For this review, take the finished solid that the model builds, in its own axes (mm). A direction names the side the tool comes from. Round coordinates to 2 decimals unless told otherwise and drop trailing zeros. Write each loop counter-clockwise with the first axis right and the second up, starting at its lowest first coordinate (ties: lowest second). Pieces come first, ordered by that corner, then holes. Notation, with made-up numbers: (46, -6) - (54, -6) arc R23 ccw to (54, 18) - close; hole circle Ø2 at (15.5, 68.25). An arc over 180 degrees is marked (long way). One line per item, written item: value. Start each with the question number.
Q1. Tool access review of faces 4 (the face through (-2.019, -46, 3)), 5 (the face through (24.11, -21.92, 2.96)), 6 (the face through (21.81, -25.64, 2.96)): name each direction out of +Z, -Z, +X, -X, +Y, -Y from which nothing blocks a thin tool from reaching the whole face with its end or side.
Q2. For probe 1 along Y at (x, z) = (-6, 1.75); probe 2 along X at (y, z) = (-29.5, 3.25); probe 3 along X at (y, z) = (-23.25, 2.2), list the stretches that pass through material, from the lowest coordinate up.
Q3. Add section A-A on x = 25. Write out the cut boundary in (y, z), and give its area (3 significant figures).
Q4. Add section B-B on z = 0.6. Give the number of separate pieces and of enclosed holes in the cut face, and give its area (3 significant figures).
Q5. Add section D-D on x = 9. Write out the cut boundary in (y, z), and give its area (3 significant figures).
Q6. Clearance check with flat-ended pins moving along their axes: pin 1 Ø2.5 at (x, y) = (25.18, -44.68) entering from -Z; pin 2 Ø4 at (x, y) = (4, -26) entering from +Z. State where each tip first meets the part, or that it passes through.
Q7. Add section C-C on y = -38. Write out the cut boundary in (x, z).
Q8. Mouldability with a two-part tool opening along Y and no side actions: class faces 1 (the face through (-1.449, -41.785, 2.958)), 2 (the face through (10, -34, 0)), 3 (the face through (1.5, -30.38, 2.96)) as +Y half, -Y half, draft (parallel to the pull), parting line (faces both ways), or undercut.
Autodesk Inventor part; units mm, degrees
ref_plane "YZ Plane" through (0, 0, 0) normal (1, 0, 0) x (0, 1, 0)
ref_plane "XZ Plane" through (0, 0, 0) normal (0, 1, 0) x (-1, 0, 0)
ref_plane "XY Plane" through (0, 0, 0) normal (0, 0, 1) x (1, 0, 0)
sketch "스케치1" plane through (0, 0, 0) normal (0, 0, 1) x (1, 0, 0)
  line L0 (22.3806, -23.2436) -> (22.3806, 15.7564)
  arc A0 (20.3806, -26.2436) -> (22.3806, -24.2436) centre (20.3806, -24.2436) ccw
  line L1 (22.3806, -24.2436) -> (22.3806, -22.8439)
  line L2 (18.7808, -26.2436) -> (20.3806, -26.2436)
  line L3 (0.9806, -26.2436) -> (19.3806, -26.2436)
  arc A1 (-2.0194, -24.2436) -> (-0.0194, -26.2436) centre (-0.0194, -24.2436) ccw
  line L4 (-0.0194, -26.2436) -> (1.5803, -26.2436)
  line L5 (-2.0194, -24.2436) -> (-2.0194, -22.8439)
  line L6 (-2.0194, 15.7564) -> (-2.0194, -23.2436)
  circle A2 centre (25.1806, -22.7436) radius 1.45
  circle A3 centre (18.6806, -29.0436) radius 1.45
  circle A4 centre (1.6806, -29.0436) radius 1.45
  circle A5 centre (-4.8194, -22.7436) radius 1.45
  line L7 (-7.6194, -18.7138) -> (27.9806, -18.7138)
  line L8 (-7.6194, -18.7138) -> (27.9806, -18.7138)
  arc A6 (-0.0194, -41.1839) -> (-2.0194, -43.1839) centre (-0.0194, -43.1839) ccw
  line L9 (-2.0194, -43.1839) -> (-2.0194, -44.5837)
  line L10 (1.5803, -41.1839) -> (-0.0194, -41.1839)
  line L11 (19.3806, -41.1839) -> (0.9806, -41.1839)
  arc A7 (22.3806, -43.1839) -> (20.3806, -41.1839) centre (20.3806, -43.1839) ccw
  line L12 (20.3806, -41.1839) -> (18.7808, -41.1839)
  line L13 (22.3806, -43.1839) -> (22.3806, -44.5837)
  circle A8 centre (-4.8194, -44.6839) radius 1.45
  circle A9 centre (1.6806, -38.3839) radius 1.45
  circle A10 centre (18.6806, -38.3839) radius 1.45
  circle A11 centre (25.1806, -44.6839) radius 1.45
  line L14 (27.9806, -48.7138) -> (-7.6194, -48.7138)
  line L15 (27.9806, -48.7138) -> (-7.6194, -48.7138)
  line L16 (-2.0194, -44.5837) -> (-2.0194, -48.7138)
  line L17 (22.3806, -44.5837) -> (22.3806, -48.7138)
  line L18 (10.1806, -18.7138) -> (10.1806, -33.7138)
  line L19 (-7.6194, -48.7138) -> (27.9806, -48.7138)
  line L20 (27.9806, -48.7138) -> (27.9806, -33.7138)
  line L21 (27.9806, -33.7138) -> (-7.6194, -33.7138)
  line L22 (-7.6194, -33.7138) -> (-7.6194, -48.7138)
  circle A12 centre (10.1806, -33.7138) radius 2.4281
  line L23 (-7.6194, -18.7138) -> (-7.6194, -34.6206)
  line L24 (27.9806, -18.7138) -> (27.9806, -33.7138)
  circle A13 centre (-4.8194, -22.7436) radius 1.35
  circle A14 centre (1.6806, -29.0436) radius 1.35
  circle A15 centre (18.6806, -29.0436) radius 1.35
  circle A16 centre (25.1806, -22.7436) radius 1.35
  circle A17 centre (18.6806, -38.3839) radius 1.35
  circle A18 centre (25.1806, -44.6839) radius 1.35
  circle A19 centre (1.6806, -38.3839) radius 1.35
  circle A20 centre (-4.8194, -44.6839) radius 1.35
  point P0 (0, 0)
  point P1 (-7.1939, 58.7329)
  point P2 (22.3806, -18.7138)
  point P3 (-2.0194, -18.7138)
  point P4 (27.9806, -25.8436)
  point P5 (-7.6194, -25.8436)
  point P6 (-2.0194, -44.1839)
  point P7 (-7.6194, -41.5839)
  point P8 (22.3806, -44.1839)
  point P9 (27.9806, -41.5839)
  point P10 (-2.0194, -18.7138)
  point P11 (22.3806, -18.7138)
  point P12 (10.1806, -48.7138)
  dimension "d11" = 30
  dimension "d12" = 15
  dimension "d13" = 15
  dimension "d14" = 2.7
  dimension "d15" = 2.7
  dimension "d16" = 2.7
  dimension "d17" = 2.7
  dimension "d18" = 2.7
  dimension "d19" = 2.7
  dimension "d20" = 2.7
  dimension "d21" = 2.7
extrude "돌출1" add sketch "스케치1" along normal blind 6 contours L0 L7 L24 L21 A12 L18 L3 L2 A0 L1 | L6 L5 A1 L4 L3 L18 A12 L21 L23 L7 | L20 L14 L17 L13 A7 L12 L11 L10 A6 L9 L16 L22 L21 A12 | A12 L21 L18 | L18 L21 A12 | A12 L21 | A2 | A3 | A4 | A5 | A8 | A9 | A10 | A11
properties part number "frame_arm_to_hand1" material "PMMA 플라스틱"
Result set:
1. face 4: +Z, -Z, -Y
1. face 5: +Z, -Z
1. face 6: +Z, -Z, +Y
2. probe 1: y = -48.71 to -45.34, -44.03 to -23.4, -22.09 to -18.71
2. probe 2: x = -7.62 to 0.41, 2.95 to 17.41, 19.95 to 27.98
2. probe 3: x = -7.62 to -6.07, -3.57 to -2.02, 22.38 to 23.93, 26.43 to 27.98
3. outline: (-48.71, 0) - (-46.02, 0) - (-46.02, 6) - (-48.71, 6) - close; (-43.35, 0) - (-24.08, 0) - (-24.08, 6) - (-43.35, 6) - close; (-21.41, 0) - (-18.71, 0) - (-18.71, 6) - (-21.41, 6) - close
3. area: 148 mm^2
4. separate pieces: 1
4. enclosed holes: 8
4. area: 658 mm^2
5. outline: (-41.18, 0) - (-26.24, 0) - (-26.24, 6) - (-41.18, 6) - close
5. area: 89.6 mm^2
6. pin 1: passes through
6. pin 2: stops at z = 6
7. outline: (-7.62, 0) - (0.39, 0) - (0.39, 6) - (-7.62, 6) - close; (2.97, 0) - (17.39, 0) - (17.39, 6) - (2.97, 6) - close; (19.97, 0) - (27.98, 0) - (27.98, 6) - (19.97, 6) - close
8. face 1: -Y half
8. face 2: draft
8. face 3: undercut
